Here's how the part is built. I have some questions about the finished solid (model axes, mm). Face numbers are marked on the shaded views. A direction names the side the tool comes from. Coordinates: 2 decimals unless noted, no trailing zeros. Write each loop counter-clockwise with the first axis right and the second up, starting at its lowest first coordinate (ties: lowest second). Pieces come first, ordered by that corner, then holes.
(1) Imagine slicing it at C-C, the plane x = -9.75. List the corners of the cut face in (y, z) for me, plus the area to 3 significant figures.
(2) For pin 1 Ø4.5 at (x, y) = (8.49, -8.49) entering from +Z; pin 2 Ø6.5 at (x, y) = (-8, 7) entering from -Z; pin 3 Ø5 at (x, y) = (-8.5, -8.5) entering from -Z; pin 4 Ø6 at (y, z) = (7.5, 14) entering from +X, each with a flat end and sliding along its axis, tell me the tip position at first contact or that it passes through.
(3) Imagine slicing it at D-D, the plane z = 8. List the corners of the cut face in (x, y) for me, plus the area to 3 significant figures.
(4) Which directions (+Z, -Z, +X, -X, +Y, -Y) give clear straight access to the entire face, cutting with the end or side of a thin tool? Please do the marked faces 1, 2 and 3.
(5) Thinking about a two-plate mould opening in Y: for the marked faces 4, 5, 6 and 7, which applies, released by +Y, released by -Y, zero draft, split by the parting line, or undercut?
(6) Imagine slicing it at A-A, the plane y = 0. List the corners of the cut face in (x, z) for me.
(7) Please list where these lines run through material, in increasing order: probe 1 along Y at (x, z) = (7, 1); probe 2 along Z at (x, y) = (11, 8.5); probe 3 along Y at (x, z) = (1, 12.5).
```python
from build123d import *

# Parameters (mm, degrees)
SKETCH_1_R          = 4
SKETCH_1_R_2        = 3
SKETCH_1_R_3        = 1.75
EXTRUDE_1_DEPTH     = 4
SKETCH_1_3_R        = 3
SKETCH_1_3_R_2      = 1.75
CUT_EXTRUDE_1_DEPTH = 3.1
SKETCH_2_R          = 7.5
SKETCH_2_R_2        = 4
EXTRUDE_2_DEPTH     = 12
CHAMFER_1_SIZE      = 0.5
CHAMFER_2_SIZE      = 0.5
FILLET_1_R          = 0.5


with BuildPart() as part:
    # Sketch 1 → Extrude 1 (new body)
    # profile 1 of 5: a face of its own
    with BuildSketch(Plane.XY):
        Polygon((10.5, 12.5), (12.5, 10.5), (12.5, -10.5), (10.5, -12.5), (-10.5, -12.5), (-12.5, -10.5), (-12.5, 10.5), (-10.5, 12.5), align=None)
        Circle(SKETCH_1_R, mode=Mode.SUBTRACT)
        with Locations((8.485281374, 8.485281374)):
            Circle(SKETCH_1_R_2, mode=Mode.SUBTRACT)
        with Locations((8.485281374, -8.485281374)):
            Circle(SKETCH_1_R_2, mode=Mode.SUBTRACT)
        with Locations((-8.485281374, -8.485281374)):
            Circle(SKETCH_1_R_2, mode=Mode.SUBTRACT)
        with Locations((-8.485281374, 8.485281374)):
            Circle(SKETCH_1_R_2, mode=Mode.SUBTRACT)
    # profile 2 of 5: a face of its own
    with BuildSketch(Plane.XY):
        with Locations((-8.485281374, 8.485281374)):
            Circle(SKETCH_1_R_2)
        with Locations((-8.485281374, 8.485281374)):
            Circle(SKETCH_1_R_3, mode=Mode.SUBTRACT)
    # profile 3 of 5: a face of its own
    with BuildSketch(Plane.XY):
        with Locations((8.485281374, 8.485281374)):
            Circle(SKETCH_1_R_2)
        with Locations((8.485281374, 8.485281374)):
            Circle(SKETCH_1_R_3, mode=Mode.SUBTRACT)
    # profile 4 of 5: a face of its own
    with BuildSketch(Plane.XY):
        with Locations((-8.485281374, -8.485281374)):
            Circle(SKETCH_1_R_2)
        with Locations((-8.485281374, -8.485281374)):
            Circle(SKETCH_1_R_3, mode=Mode.SUBTRACT)
    # profile 5 of 5: a face of its own
    with BuildSketch(Plane.XY):
        with Locations((8.485281374, -8.485281374)):
            Circle(SKETCH_1_R_2)
        with Locations((8.485281374, -8.485281374)):
            Circle(SKETCH_1_R_3, mode=Mode.SUBTRACT)
    extrude(amount=EXTRUDE_1_DEPTH)

    # Sketch 1_3 → Cut-Extrude 1 (cut)
    # profile 1 of 4: a face of its own
    with BuildSketch(Plane.XY):
        with Locations(Location((8.485281374, -8.485281374, 0), (0, 0, 180))):
            Circle(SKETCH_1_3_R)
        with Locations((8.485281374, -8.485281374)):
            Circle(SKETCH_1_3_R_2, mode=Mode.SUBTRACT)
    # profile 2 of 4: a face of its own
    with BuildSketch(Plane.XY):
        with Locations(Location((-8.485281374, -8.485281374, 0), (0, 0, 180))):
            Circle(SKETCH_1_3_R)
        with Locations((-8.485281374, -8.485281374)):
            Circle(SKETCH_1_3_R_2, mode=Mode.SUBTRACT)
    # profile 3 of 4: a face of its own
    with BuildSketch(Plane.XY):
        with Locations(Location((-8.485281374, 8.485281374, 0), (0, 0, 180))):
            Circle(SKETCH_1_3_R)
        with Locations((-8.485281374, 8.485281374)):
            Circle(SKETCH_1_3_R_2, mode=Mode.SUBTRACT)
    # profile 4 of 4: a face of its own
    with BuildSketch(Plane.XY):
        with Locations(Location((8.485281374, 8.485281374, 0), (0, 0, 180))):
            Circle(SKETCH_1_3_R)
        with Locations((8.485281374, 8.485281374)):
            Circle(SKETCH_1_3_R_2, mode=Mode.SUBTRACT)
    extrude(amount=CUT_EXTRUDE_1_DEPTH, mode=Mode.SUBTRACT)

    # Sketch 2 → Extrude 2 (add)
    with BuildSketch(Plane.XY.offset(4)):
        Circle(SKETCH_2_R)
        Circle(SKETCH_2_R_2, mode=Mode.SUBTRACT)
    extrude(amount=EXTRUDE_2_DEPTH)

    # Chamfer 1
    chamfer_1_edges = [part.edges().sort_by_distance(p)[0] for p in [
        (-7.5, 0, 16),
    ]]
    chamfer(chamfer_1_edges, length=CHAMFER_1_SIZE)

    # Chamfer 2
    chamfer_2_edges = [part.edges().sort_by_distance(p)[0] for p in [
        (12.5, 0, 0),
        (11.5, -11.5, 0),
        (0, -12.5, 0),
        (-11.5, -11.5, 0),
        (-12.5, 0, 0),
        (-11.5, 11.5, 0),
        (0, 12.5, 0),
        (11.5, 11.5, 0),
    ]]
    chamfer(chamfer_2_edges, length=CHAMFER_2_SIZE)

    # Fillet 1
    fillet_1_edges = [part.edges().sort_by_distance(p)[0] for p in [
        (11.5, 11.5, 4),
        (0, 12.5, 4),
        (-11.5, 11.5, 4),
        (-12.5, 0, 4),
        (-11.5, -11.5, 4),
        (0, -12.5, 4),
        (11.5, -11.5, 4),
        (12.5, 0, 4),
    ]]
    fillet(fillet_1_edges, radius=FILLET_1_R)


solid = part.part
```
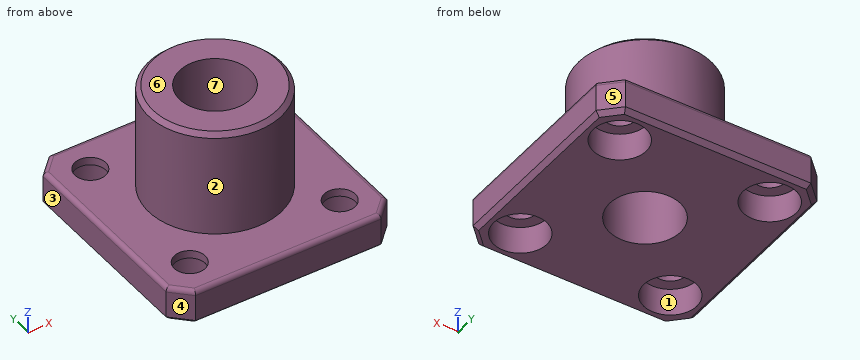
Recorded:
1. outline: (-12.5, 0.5) - (-12, 0) - (-11.21, 0) - (-11.21, 3.1) - (-9.69, 3.1) - (-9.69, 4) - (-12, 4) arc R0.5 ccw to (-12.5, 3.5) - close; (-7.28, 3.1) - (-5.76, 3.1) - (-5.76, 0) - (5.76, 0) - (5.76, 3.1) - (7.28, 3.1) - (7.28, 4) - (-7.28, 4) - close; (9.69, 3.1) - (11.21, 3.1) - (11.21, 0) - (12, 0) - (12.5, 0.5) - (12.5, 3.5) arc R0.5 ccw to (12, 4) - (9.69, 4) - close
1. area: 61.6 mm2
2. pin 1: stops at z = 4
2. pin 2: stops at z = 0
2. pin 3: stops at z = 3.1
2. pin 4: stops at x = 6
3. outline: circle Ø15 at (0, 0); hole circle Ø8 at (0, 0)
3. area: 126 mm2
4. face 1: -Z
4. face 2: +Z
4. face 3: +Z, -Z, -X, +Y, -Y
5. face 4: released by -Y
5. face 5: released by +Y
5. face 6: zero draft
5. face 7: undercut
6. outline: (-12.5, 0.5) - (-12, 0) - (-4, 0) - (-4, 16) - (-7, 16) - (-7.5, 15.5) - (-7.5, 4) - (-12, 4) arc R0.5 ccw to (-12.5, 3.5) - close; (4, 0) - (12, 0) - (12.5, 0.5) - (12.5, 3.5) arc R0.5 ccw to (12, 4) - (7.5, 4) - (7.5, 15.5) - (7, 16) - (4, 16) - close
7. probe 1: y = -12.5 to -11.09, -5.88 to 5.88, 11.09 to 12.5
7. probe 2: z = 3.1 to 4
7. probe 3: y = -7.43 to -3.87, 3.87 to 7.43
